For this review, take the finished solid that the model builds, in its own axes (mm). A direction names the side the tool comes from. Round coordinates to 2 decimals unless told otherwise and drop trailing zeros. Loops run counter-clockwise (first coordinate to the right, second up) from the corner with the lowest first, then second, coordinate; pieces in that order, holes last. Notation, with made-up numbers: M -36,-25 L 7,-25 A27 ccw 7,-7 Z; hole C 88,17.5 d1. An arc over 180 degrees is marked long. One line per question, with ' | ' between items. Start each with the question number.
1) We need section C-C (z = 1.4). Give the boundary of the cut face in (x, y) (3 decimals), and give its area (3 significant figures).
2) For probe 1 along Y at (x, z) = (1.25, 0.65); probe 2 along X at (y, z) = (0, 0.95) (3 decimals); probe 3 along X at (y, z) = (0, 0.8) (3 decimals), list the stretches that pass through material, from the lowest coordinate up. Write a range as from..to.
3) For pin 1 Ø1.5 at (x, y) = (-0.5, 1) entering from +Z; pin 2 Ø1 at (x, z) = (0, 1.5) entering from +Y (3 decimals), all flat-tipped, find the tip position at first contact; note any pin that passes through.
4) We need section B-B (z = 0.45). Give the boundary of the cut face in (x, y) (3 decimals), and give its area (3 significant figures).
5) We need section A-A (z = -0.2). Give the boundary of the cut face in (x, y), and give its area (3 significant figures).
6) For faces 1 (the face through (1.947, 3.437, -0.238)), 2 (the face through (-3, -0.67, 0.3)), 3 (the face through (-3.588, -0.797, 1.454)), list the 3-axis set-ups (+Z, -Z, +X, -X, +Y, -Y) from which the entire face can be reached by the end or side of a thin tool; tool diameter is ignored.
7) Mouldability with a two-part tool opening along Y and no side actions: class faces 4 (the face through (2.003, -3.405, -0.238)), 5 (the face through (-3.544, 2.058, -0.546)), 6 (the face through (2, 0, 1)) as pulls with the +Y half, pulls with the -Y half, needs draft (parallel to the pull), parting line crosses it, or undercut.
```python
from build123d import *

# Parameters (mm, degrees)
BOSS_EXTRUDE1_DEPTH = 0.6
SKETCH6_W           = 2.3
SKETCH6_H           = 2


with BuildPart() as part:
    # Sketch1 → Revolve1 (revolve)
    with BuildSketch(Plane.ZY):
        Polygon((0, 3.075), (0.6, 3.075), (1.2, 3.675), (1.7, 3.675), (1.7, 0), (0, 0), (-0.6, 0), (-0.6, 3.95), (0, 3.95), align=None)
    revolve(axis=Axis((0, 0, 1.7), (0, 0, -1)))

    # Sketch3 → Boss-Extrude1 (add)
    with BuildSketch(Plane(origin=(0, 0, -0.6), x_dir=(-1, 0, 0), z_dir=(0, 0, -1))):
        Polygon((0, 4.561067127), (-3.95, 2.280533563), (-3.95, -2.280533563), (0, -4.561067127), (3.95, -2.280533563), (3.95, 2.280533563), align=None)
    extrude(amount=-BOSS_EXTRUDE1_DEPTH)

    # Sketch10 → Cut-Revolve4 (revolve, cut)
    with BuildSketch(Plane(origin=(0, 0, 0), x_dir=(0, 0, -1), z_dir=(1, 0, 0))):
        Polygon((0.377589755, 4.561067127), (0.6, 4.561067127), (0.6, 3.95), align=None)
    revolve(axis=Axis((0, 0, -0.6), (0, 0, 1)), mode=Mode.SUBTRACT)

    # Sketch6 → Cut-Revolve2 (revolve, cut)
    with BuildSketch(Plane(origin=(0, 0, 0), x_dir=(0, 0, -1), z_dir=(1, 0, 0))):
        with Locations((-0.55, 1)):
            Rectangle(SKETCH6_W, SKETCH6_H)
    revolve(axis=Axis((0, 0, -0.6), (0, 0, 1)), mode=Mode.SUBTRACT)


solid = part.part
```
Answers below:
1) outline: C 0,0 d7.35; hole C 0,0 d4 | area: 29.9 mm^2
2) probe 1: -2.86..-1.56, 1.56..2.86 | probe 2: -3.425..-2, 2..3.425 | probe 3: -3.275..-2, 2..3.275
3) pin 1: through | pin 2: y = 3.675
4) outline: C 0,0 d6.15; hole C 0,0 d4 | area: 17.1 mm^2
5) outline: M -3.95,-2.28 L 0,-4.56 L 3.95,-2.28 L 3.95,2.28 L 0,4.56 L -3.95,2.28 Z; hole C 0,0 d4 | area: 41.5 mm^2
6) face 1: +Z, -Z, +X, +Y | face 2: none | face 3: +Z
7) face 4: pulls with the -Y half | face 5: pulls with the +Y half | face 6: undercut
